from build123d import *

# Parameters (mm, degrees)
BODY_DEPTH   = 71.42
POCKET_DEPTH = 62.42
SKETCH3_R    = 4.2
HOLESX_DEPTH = 6.35
SKETCH4_R    = 4.2
HOLESY_DEPTH = 6.35


with BuildPart() as part:
    # Sketch1 → Body (new body)
    with BuildSketch(Plane.XY.offset(-35.71)):
        Polygon((0, 0), (38.1, 0), (38.1, 6.35), (6.35, 38.1), (0, 38.1), align=None)
    extrude(amount=BODY_DEPTH)

    # Sketch2 → Pocket (cut)
    with BuildSketch(Plane.XY.offset(31.21)):
        Polygon((6.35, 6.35), (48.1, 6.35), (6.35, 48.1), align=None)
    extrude(amount=-POCKET_DEPTH, mode=Mode.SUBTRACT)

    # Sketch3 → HolesX (cut)
    with BuildSketch(Plane(origin=(0, 6.35, 0), x_dir=(1, 0, 0), z_dir=(0, 1, 0))):
        with Locations(Location((19.05, 19.05, 0), (0, 0, 270))):
            Circle(SKETCH3_R)
        with Locations(Location((19.05, -19.05, 0), (0, 0, 270))):
            Circle(SKETCH3_R)
    extrude(amount=-HOLESX_DEPTH, mode=Mode.SUBTRACT)

    # Sketch4 → HolesY (cut)
    with BuildSketch(Plane(origin=(6.35, 0, 0), x_dir=(0, 0, -1), z_dir=(1, 0, 0))):
        with Locations((19.05, 19.05)):
            Circle(SKETCH4_R)
        with Locations((-19.05, 19.05)):
            Circle(SKETCH4_R)
    extrude(amount=-HOLESY_DEPTH, mode=Mode.SUBTRACT)


solid = part.part
Design review of the part built by this model. Coordinates are the model's own, in mm. A direction names the side the tool comes from. Coordinates: 2 decimals unless noted, no trailing zeros. Loops run counter-clockwise (first coordinate to the right, second up) from the corner with the lowest first, then second, coordinate; pieces in that order, holes last. Notation, with made-up numbers: M 52.5,-13.5 L 86.5,-13.5 A31 cw 86.5,22.5 Z; hole C -27.75,31 d5. An arc over 180 degrees is marked long. Answer as CSV lines item,"result".
Item 1: For probe 1 along Z at (x, y) = (3.5, 19); probe 2 along X at (y, z) = (3, -19), list the stretches that pass through material, from the lowest coordinate up.
Answer list:
probe 1,"-35.71 to -23.25, -14.85 to 14.85, 23.25 to 35.71"
probe 2,"0 to 14.85, 23.25 to 38.1"
Item 2: The part is to be moulded in two halves that separate along X. For faces 1 (the face through (3.22, 14.95, 19.96)), 2 (the face through (14.95, 3.22, -19.96)), 3 (the face through (14.95, 3.22, 18.14)), 4 (the face through (6.35, 22, 0)), say which applies: pulls with the +X half, pulls with the -X half, needs draft (parallel to the pull), parting line crosses it, or undercut.
Answer list:
face 1,"needs draft"
face 2,"undercut"
face 3,"undercut"
face 4,"pulls with the +X half"
Item 3: Add section A-A on y = 19.05. State the section outline as (x, z) points.
Answer list:
outline,"M 0,-35.71 L 25.4,-35.71 L 25.4,-31.21 L 6.35,-31.21 L 6.35,-23.25 L 0,-23.25 Z; M 0,-14.85 L 6.35,-14.85 L 6.35,14.85 L 0,14.85 Z; M 0,23.25 L 6.35,23.25 L 6.35,31.21 L 25.4,31.21 L 25.4,35.71 L 0,35.71 Z"
Item 4: Add section B-B on z = -19.05. State the section outline as (x, y) points, plus the area to 3 significant figures.
Answer list:
outline,"M 0,0 L 14.85,0 L 14.85,6.35 L 6.35,6.35 L 6.35,14.85 L 0,14.85 Z; M 0,23.25 L 6.35,23.25 L 6.35,38.1 L 0,38.1 Z; M 23.25,0 L 38.1,0 L 38.1,6.35 L 23.25,6.35 Z"
area,"337 mm²"
Item 5: Add section D-D on y = 14. State the section outline as (x, z) points, plus the area to 3 significant figures.
Answer list:
outline,"M 0,-35.71 L 30.45,-35.71 L 30.45,-31.21 L 6.35,-31.21 L 6.35,31.21 L 30.45,31.21 L 30.45,35.71 L 0,35.71 Z"
area,"670 mm²"
Item 6: For P1, Ø4, axis at y = 16.5, z = -4.5, coming from the +X side, flat-tipped, find the tip position at first contact; note if it passes through.
Answer list:
P1,"x = 6.35"
Item 7: Machinability: for faces 5 (the face through (19, 0, 0)), 6 (the face through (22, 6.35, 0)), which of the approach directions +Z, -Z, +X, -X, +Y, -Y give a long, thin tool a straight path to every point of the face, cutting with its end or side? Answer none if there is none.
Answer list:
face 5,"+Z, -Z, +X, -X, -Y"
face 6,"+X, +Y"
